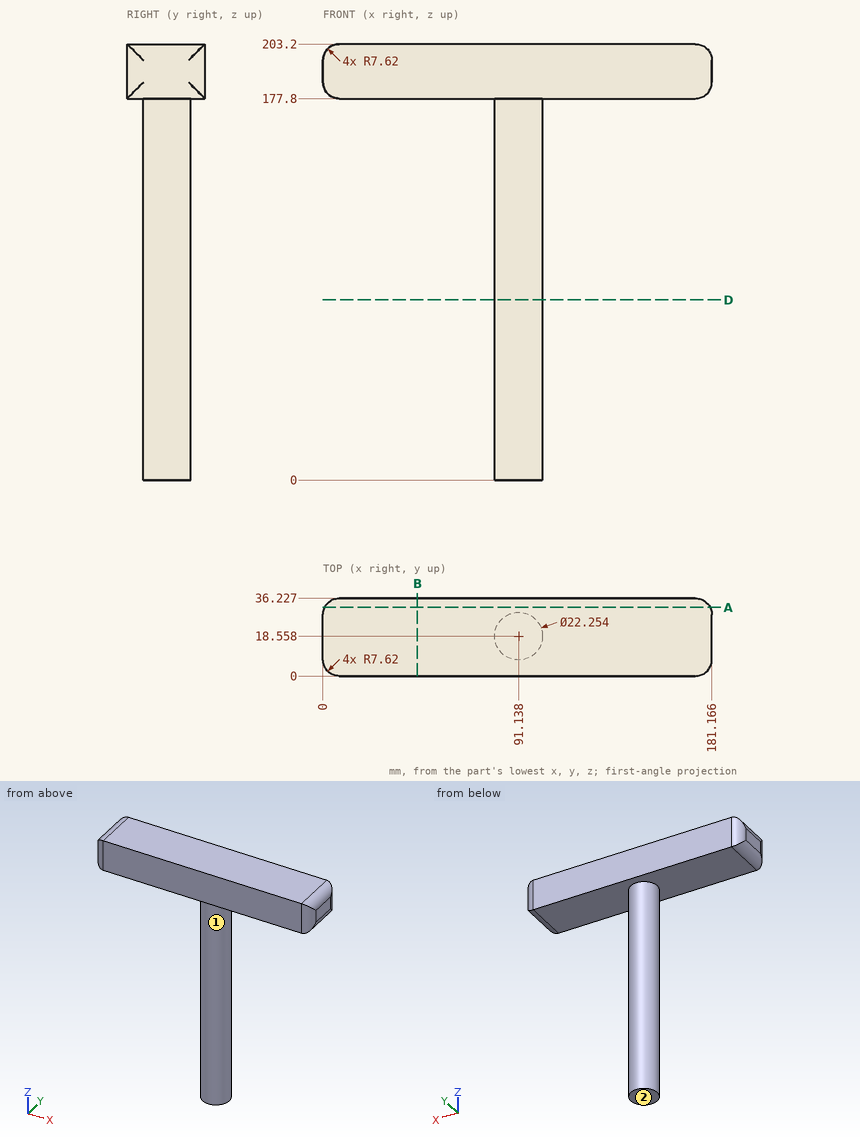
Print and shaded views of the part. All mm, measured from the part's lowest x, y and z. A direction names the side the tool comes from. Give positions to 0.01 mm unless a question says otherwise; leave off trailing zeros. Order: outer loops, then holes, each group sorted by start corner. A loop starts at its lowest first (then second) coordinate and runs counter-clockwise, first axis right, second up. Notation, with made-up numbers: (-9, 33) - (2, 33) arc R18 ccw to (2, 59) - close; hole circle Ø9 at (89.5, 56). An arc over 180 degrees is marked (long way). Use a Markdown table: item, result.
1) Flat gauge pin, fed straight in: P1, Ø2, axis at y = 29, z = 58, coming from the +X side (1 decimal). Where does the tip first touch, or does it go through?
Checked values:
| item | result |
|---|---|
| P1 | x = 97 |
2) 3-axis set-ups, long thin cutter, end or side, ignore diameter. For the marked faces 1 and 2: which of +Z, -Z, +X, -X, +Y, -Y reach the whole face in a straight line?
Checked values:
| item | result |
|---|---|
| face 1 | -Z |
| face 2 | -Z, +X, -X, +Y, -Y |
3) Saw through at B-B on x = 44. List the corners of the cut face in (y, z).
Checked values:
| item | result |
|---|---|
| outline | (0, 177.8) - (36.23, 177.8) - (36.23, 203.2) - (0, 203.2) - close |
4) Saw through at D-D on z = 84. List the corners of the cut face in (x, y) (1 decimal), plus the area to 3 significant figures.
Checked values:
| item | result |
|---|---|
| outline | circle Ø22.3 at (91.1, 18.6) |
| area | 389 mm² |
5) Probe L1, parallel to Z at x = 96, y = 33.5; L2, parallel to X at y = 18.5, z = 159.5 (1 decimal); L3, parallel to X at y = 9, z = 44.5 (1 decimal). List the from-to ranges inside material, lowest first. Write a range as from..to.
Checked values:
| item | result |
|---|---|
| L1 | 177.8..203.2 |
| L2 | 80..102.3 |
| L3 | 85.4..96.8 |
6) Saw through at A-A on y = 32. List the corners of the cut face in (x, z) (1 decimal), plus the area to 3 significant figures.
Checked values:
| item | result |
|---|---|
| outline | (0.8, 182) arc R7.6 ccw to (7.6, 177.8) - (173.5, 177.8) arc R7.6 ccw to (180.4, 182) - (180.4, 199) arc R7.6 ccw to (173.5, 203.2) - (7.6, 203.2) arc R7.6 ccw to (0.8, 199) - close |
| area | 4,530 mm² |
